Work out the finished part from the listing and answer in its coordinate system (mm). Coordinates: 2 decimals unless noted, no trailing zeros. Write each loop counter-clockwise with the first axis right and the second up, starting at its lowest first coordinate (ties: lowest second). Pieces come first, ordered by that corner, then holes. Notation, with made-up numbers: (8.25, -31) - (25.25, -31) arc R19 ccw to (25.25, -4) - close; hole circle Ø4 at (-5.5, 77). An arc over 180 degrees is marked (long way). One line per item, written item: value.
```python
from build123d import *

# Parameters (mm, degrees)
SKETCH1_R                           = 2.5
BOSS_EXTRUDE1_DEPTH                 = 13
M2X0_4_TAPPED_HOLE1_D               = 1.6
M2X0_4_TAPPED_HOLE1_DEPTH           = 5.2
M2X0_4_TAPPED_HOLE1_TIP             = 0.480688495
M2X0_4_TAPPED_HOLE1_ON_FACE_2_D     = 1.6
M2X0_4_TAPPED_HOLE1_ON_FACE_2_DEPTH = 5.2
M2X0_4_TAPPED_HOLE1_ON_FACE_2_TIP   = 0.480688495


with BuildPart() as part:
    # Sketch1 → Boss-Extrude1 (new, symmetric)
    with BuildSketch(Plane(origin=(0, 0, 0), x_dir=(1, 0, 0), z_dir=(0, 1, 0))):
        with Locations(Location((0, 0, 0), (0, 0, 90))):
            Circle(SKETCH1_R)
    extrude(amount=BOSS_EXTRUDE1_DEPTH, both=True)

    # M2x0.4 Tapped Hole1
    with Locations(Plane.ZX.offset(13)):
        with Locations((0, 0)):
            Hole(M2X0_4_TAPPED_HOLE1_D / 2, depth=M2X0_4_TAPPED_HOLE1_DEPTH)
            with Locations((0, 0, -(M2X0_4_TAPPED_HOLE1_DEPTH + M2X0_4_TAPPED_HOLE1_TIP / 2))):  # 118° drill point
                Cone(0, M2X0_4_TAPPED_HOLE1_D / 2, M2X0_4_TAPPED_HOLE1_TIP, mode=Mode.SUBTRACT)

    # M2x0.4 Tapped Hole1 on face 2
    with Locations(Plane(origin=(0, -13, 0), x_dir=(0, 0, -1), z_dir=(0, -1, 0))):
        with Locations((0, 0)):
            Hole(M2X0_4_TAPPED_HOLE1_ON_FACE_2_D / 2, depth=M2X0_4_TAPPED_HOLE1_ON_FACE_2_DEPTH)
            with Locations((0, 0, -(M2X0_4_TAPPED_HOLE1_ON_FACE_2_DEPTH + M2X0_4_TAPPED_HOLE1_ON_FACE_2_TIP / 2))):  # 118° drill point
                Cone(0, M2X0_4_TAPPED_HOLE1_ON_FACE_2_D / 2, M2X0_4_TAPPED_HOLE1_ON_FACE_2_TIP, mode=Mode.SUBTRACT)


solid = part.part
```
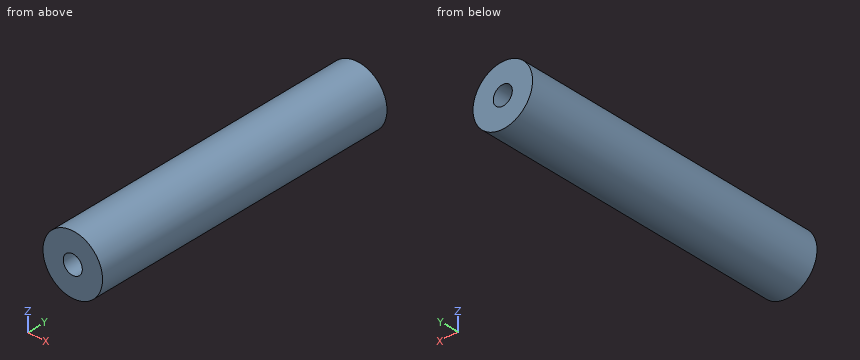
Item 1: Section A-A, the plane x = 1.5 is taken. Determine the outline of the cut face in (y, z).
Evaluation:
outline: (-13, -2) - (13, -2) - (13, 2) - (-13, 2) - close
Item 2: Given pin 1 (1.3 mm diameter, centred on x = 0, z = 0, fed in from +Y), flat-ended and moving along its own axis, determine where the tip first touches the part or whether it passes through.
Evaluation:
pin 1: stops at y = 7.71
Item 3: Section C-C, the plane z = -1.55 is taken. Determine the outline of the cut face in (x, y), then the cut area to 3 significant figures.
Evaluation:
outline: (-1.96, -13) - (1.96, -13) - (1.96, 13) - (-1.96, 13) - close
area: 102 mm2
Item 4: Consider probe 1 along X at (y, z) = (-10.95, 0); probe 2 along Z at (x, y) = (2.3, 3); probe 3 along X at (y, z) = (1.75, 0.4). Determine where each line is inside the solid, lowest interval first.
Evaluation:
probe 1: x = -2.5 to -0.8, 0.8 to 2.5
probe 2: z = -0.98 to 0.98
probe 3: x = -2.47 to 2.47
Item 5: Section B-B, the plane y = 2.5 is taken. Determine the outline of the cut face in (x, z), then the cut area to 3 significant figures.
Evaluation:
outline: circle Ø5 at (0, 0)
area: 19.6 mm2
